For this review, use the dimensioned drawing (mm, ordinates from the lowest corner) and the shaded views. Coordinates: 2 decimals unless noted, no trailing zeros. Loops run counter-clockwise (first coordinate to the right, second up) from the corner with the lowest first, then second, coordinate; pieces in that order, holes last. Notation, with made-up numbers: (69.5, 13) -> (103.5, 13) arc R29 ccw to (103.5, 42) -> close; hole circle Ø9 at (-36.5, 61.25). An arc over 180 degrees is marked (long way). One line per question, with ' | ' between items. Start each with the question number.
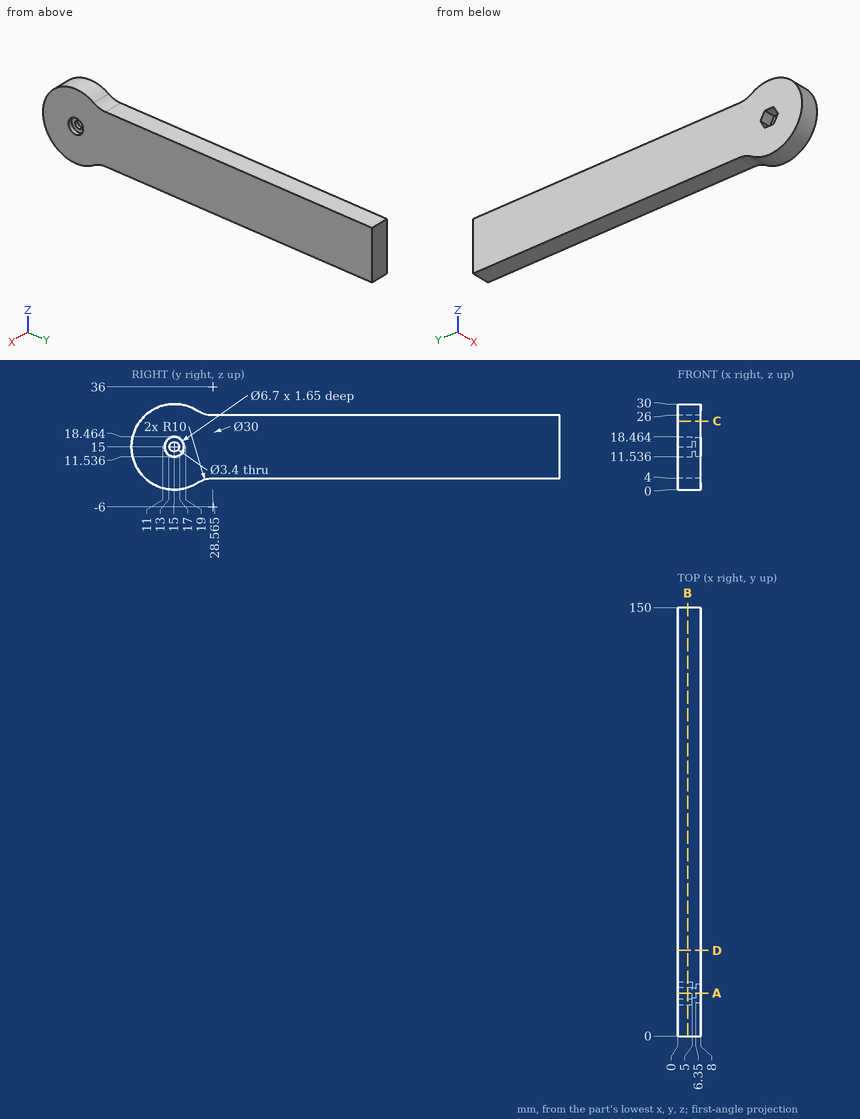
1) Consider section A-A, the plane y = 15. Write out the cut boundary in (x, z).
2) Consider section B-B, the plane x = 3.5. Write out the cut boundary in (y, z) (1 decimal), plus the area to 3 significant figures.
3) Consider section C-C, the plane z = 24. Write out the cut boundary in (x, y).
4) Insertion check: pin 1 Ø7.5 at (y, z) = (15.5, 13.5) entering from +X; pin 2 Ø1.5 at (x, z) = (2.5, 25) entering from -Y; pin 3 Ø4 at (x, y) = (4.5, 124.5) entering from +Z; pin 4 Ø4 at (y, z) = (15, 15) entering from -X. Each pin has a flat end and moves straight along its axis. Give the tip position at first contact, or say it passes through.
5) Wall thickness on L1, parallel to Y at x = 5.65, z = 15; L2, parallel to Z at x = 3.5, y = 114; L3, parallel to Y at x = 7.5, z = 15: over which ranges is each line inside the solid? List them lowest first.
6) Consider section D-D, the plane y = 30. Write out the cut boundary in (x, z), plus the area to 3 significant figures.
Filled sheet:
1) outline: (0, 0) -> (8, 0) -> (8, 11.65) -> (6.35, 11.65) -> (6.35, 13.3) -> (5, 13.3) -> (5, 11.54) -> (0, 11.54) -> close; (0, 18.46) -> (5, 18.46) -> (5, 16.7) -> (6.35, 16.7) -> (6.35, 18.35) -> (8, 18.35) -> (8, 30) -> (0, 30) -> close
2) outline: (23.1, 2.4) arc R10 cw to (28.6, 4) -> (150, 4) -> (150, 26) -> (28.6, 26) arc R10 cw to (23.1, 27.6) arc R15 ccw (long way) to start; hole (11, 15) -> (13, 11.5) -> (17, 11.5) -> (19, 15) -> (17, 18.5) -> (13, 18.5) -> close | area: 3,340 mm^2
3) outline: (0, 3) -> (8, 3) -> (8, 150) -> (0, 150) -> close
4) pin 1: x = 8 | pin 2: y = 3.19 | pin 3: z = 26 | pin 4: x = 5
5) L1: 0 to 13.3, 16.7 to 150 | L2: 4 to 26 | L3: 0 to 11.65, 18.35 to 150
6) outline: (0, 4) -> (8, 4) -> (8, 26) -> (0, 26) -> close | area: 176 mm^2
